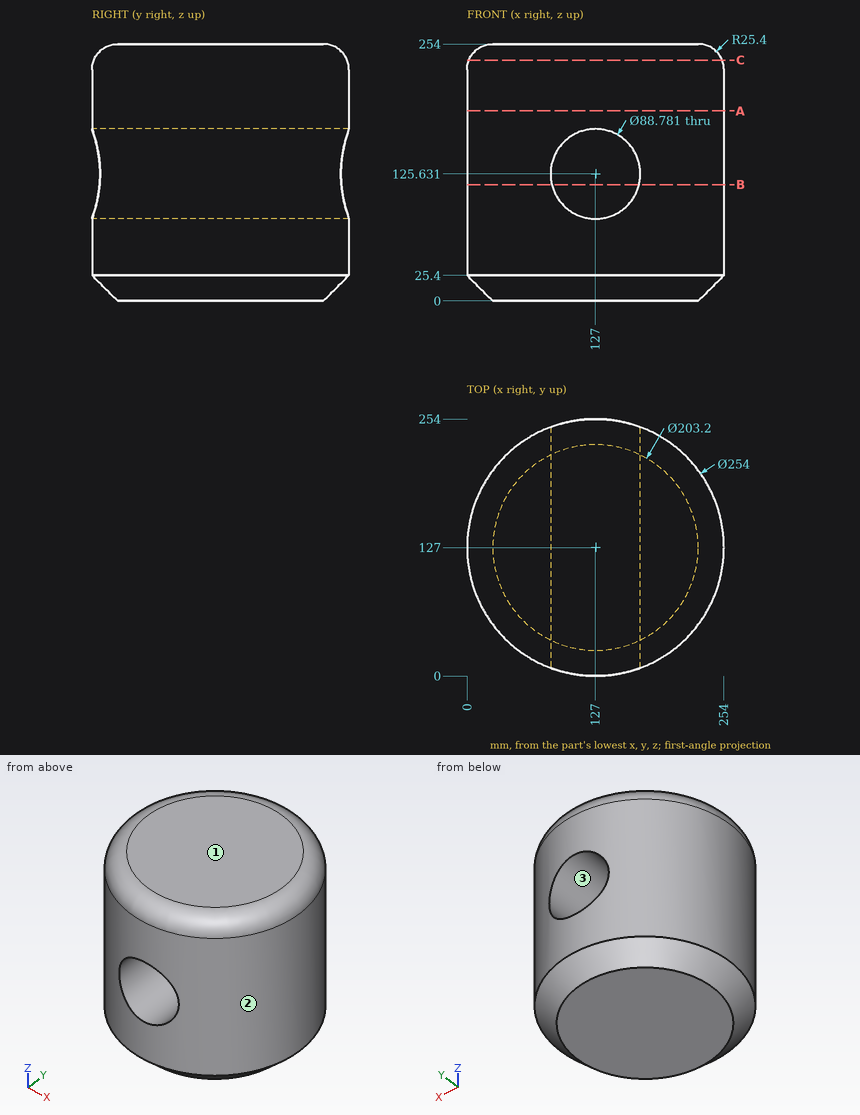
Verification items for this drawing (mm, ordinates from the low corner). Coordinates: 2 decimals unless noted, no trailing zeros. Order: outer loops, then holes, each group sorted by start corner. A loop starts at its lowest first (then second) coordinate and runs counter-clockwise, first axis right, second up. Notation, with made-up numbers: M 37.25,72 L 95.25,72 A18 ccw 95.25,90 Z; hole C 13,-26 d8. An arc over 180 degrees is marked long. One line per item, written item: value. Start each with the question number.
Item 1: Mould release check, pull along X, two halves, no side actions. Record for the marked faces 1, 2 and 3: pulls with the +X half, pulls with the -X half, needs draft (parallel to the pull), parting line crosses it, or undercut.
Item 2: Sectioned sample at A-A on z = 188. Record the cut outline in (x, y), then the cut area to 3 significant figures.
Item 3: Sectioned sample at C-C on z = 238. Record the cut outline in (x, y).
Item 4: Thickness scan on probe 1 along Z at (x, y) = (127, 144); probe 2 along Z at (x, y) = (134.5, 58); probe 3 along X at (y, z) = (119, 145). Record the ranges inside material, lowest first.
Item 5: Depth check by flat-ended pin: P1, Ø8, axis at y = 175, z = 201.5, coming from the +X side (1 decimal); P2, Ø6, axis at x = 107, z = 225.5, coming from the -Y side; P3, Ø2, axis at x = 160, z = 204.5, coming from the -Y side. Enter the tip coordinate at first touch or a pass-through.
Item 6: Sectioned sample at B-B on z = 115. Record the cut outline in (x, y).
Calculated:
1. face 1: needs draft
1. face 2: parting line crosses it
1. face 3: undercut
2. outline: C 127,127 d254
2. area: 50,700 mm^2
3. outline: C 127,127 d250.39
4. probe 1: 0 to 81.24, 170.02 to 254
4. probe 2: 0 to 81.88, 169.38 to 254
4. probe 3: 0.25 to 87.06, 166.94 to 253.75
5. P1: x = 246.1
5. P2: y = 1.14
5. P3: y = 4.1
6. outline: M 83.9,7.54 L 83.9,246.46 A127 ccw Z; M 170.1,7.54 A127 ccw 170.1,246.46 Z
